from build123d import *

# Parameters (mm, degrees)
F0_W     = 58.7917491794
F0_H     = 49.0446984768
F1_DEPTH = 40
F2_R     = 12.5
F3_DEPTH = 58.7917491794
F4_T     = -5


with BuildPart() as f1:
    # F0 (on Top) → F1 (new body)
    with BuildSketch(Plane.XY):
        with Locations((29.3958745897, 24.5223492384)):
            Rectangle(F0_W, F0_H)
    extrude(amount=F1_DEPTH)

    # F2 (on face) → F3 (cut, through all)
    with BuildSketch(Plane(origin=(0, 0, 0), x_dir=(0, -1, 0), z_dir=(-1, 0, 0))):
        with Locations((-24.5223492384, 20)):
            Circle(F2_R)
    extrude(amount=-F3_DEPTH, mode=Mode.SUBTRACT)

    # F4
    f4_openings = [f1.faces().sort_by_distance(p)[0] for p in [
        (29.395875, 24.522349, 40),
    ]]
    offset(amount=F4_T, openings=f4_openings, kind=Kind.INTERSECTION)


solid = f1.part
Source: CAD feature listing. Evaluate the final solid. Frame: model axes, mm. A direction names the side the tool comes from. Give positions to 0.01 mm unless a question says otherwise; leave off trailing zeros. Write each loop counter-clockwise with the first axis right and the second up, starting at its lowest first coordinate (ties: lowest second). Pieces come first, ordered by that corner, then holes. Notation, with made-up numbers: M -33,-4 L 21,-4 A27 cw 21,24 Z; hole C -4,34.25 d2. An arc over 180 degrees is marked long. Return JSON: item names as keys, results as strings. Group by question number.
1) Ray query, L1, parallel to X at y = 42, z = 32; L2, parallel to Y at x = 45.5, z = 35; L3, parallel to Y at x = 36.5, z = 14. Return the intervals inside material, ascending.
2) Cut plane A-A, the plane z = 20. Output: boundary loops of the cut face in (x, y), then the cut area to 3 significant figures.
3) Draft query along Z for faces 1 (the face through (29.05, 23.89, 37.49)), 2 (the face through (29, 25, 0)), 3 (the face through (29, 5, 22)). Return one class per face: released by +Z, released by -Z, zero draft, split by the parting line, or undercut.
4) Set-up query: faces 4 (the face through (29, 44.045, 22)), 5 (the face through (5, 23, 38)), 6 (the face through (28.984, 18.754, 8.91)). Return all of +Z, -Z, +X, -X, +Y, -Y with unobstructed straight access to the full face (end or side cutting, diameter ignored); none if empty.
5) Cut plane D-D, the plane z = 8.5. Output: boundary loops of the cut face in (x, y), then the cut area to 3 significant figures.
6) Cut plane B-B, the plane x = 28. Output: boundary loops of the cut face in (y, z), then the cut area to 3 significant figures.
7) Cut plane C-C, the plane y = 35. Output: boundary loops of the cut face in (x, z).
8) First-contact query: pin 1 Ø4 at (x, y) = (24.5, 17.5) entering from +Z; pin 2 Ø5 at (x, y) = (19, 18.5) entering from +Z; pin 3 Ø20 at (y, z) = (24.52, 20) entering from +X; pin 4 Ø8.5 at (x, y) = (26, 11.5) entering from +Z. Flat tips, straight axial feed; report the tip coordinate or a pass-through.
Data:
{
 "1": {"L1": "x = 0 to 5, 53.79 to 58.79", "L2": "y = 0 to 5, 15.51 to 33.54, 44.04 to 49.04", "L3": "y = 0 to 5, 8.08 to 13.56, 35.49 to 40.96, 44.04 to 49.04"},
 "2": {"outline": "M 0,0 L 58.79,0 L 58.79,12.02 L 0,12.02 Z; M 0,37.02 L 58.79,37.02 L 58.79,49.04 L 0,49.04 Z; hole M 5,5 L 53.79,5 L 53.79,7.02 L 5,7.02 Z; hole M 5,42.02 L 53.79,42.02 L 53.79,44.04 L 5,44.04 Z", "area": "1,220 mm²"},
 "3": {"face 1": "undercut", "face 2": "released by -Z", "face 3": "zero draft"},
 "4": {"face 4": "+Z", "face 5": "none", "face 6": "+X, -X"},
 "5": {"outline": "M 0,0 L 58.79,0 L 58.79,19.62 L 0,19.62 Z; M 0,29.42 L 58.79,29.42 L 58.79,49.04 L 0,49.04 Z; hole M 5,5 L 53.79,5 L 53.79,11.33 L 5,11.33 Z; hole M 5,37.71 L 53.79,37.71 L 53.79,44.04 L 5,44.04 Z", "area": "1,690 mm²"},
 "6": {"outline": "M 0,0 L 49.04,0 L 49.04,40 L 44.04,40 L 44.04,5 L 33.54,5 A17.5 ccw long 15.51,5 L 5,5 L 5,40 L 0,40 Z; hole C 24.52,20 d25", "area": "1,040 mm²"},
 "7": {"outline": "M 0,0 L 58.79,0 L 58.79,13.18 L 0,13.18 Z; M 0,26.82 L 58.79,26.82 L 58.79,40 L 53.79,40 L 53.79,34.02 L 5,34.02 L 5,40 L 0,40 Z; hole M 5,5 L 53.79,5 L 53.79,5.98 L 5,5.98 Z"},
 "8": {"pin 1": "stops at z = 36.76", "pin 2": "stops at z = 37.14", "pin 3": "passes through", "pin 4": "stops at z = 35.14"}
}
